Verification items for the finished model (mm, model axes). A direction names the side the tool comes from. Round coordinates to 2 decimals unless told otherwise and drop trailing zeros. Write each loop counter-clockwise with the first axis right and the second up, starting at its lowest first coordinate (ties: lowest second). Pieces come first, ordered by that corner, then holes. Notation, with made-up numbers: M 79,70.5 L 135,70.5 A20 cw 135,92.5 Z; hole C 14.25,26.25 d1. An arc over 180 degrees is marked long. One line per item, written item: value. Start each with the question number.
Item 1: Section check A-A, the plane y = -27.5. Record the cut outline in (x, z), then the cut area to 3 significant figures.
Item 2: Draft check along X on faces 4 (the face through (-1.671, -50.089, 3.473)), 5 (the face through (3.916, -98, 9)), 6 (the face through (2.498, -51, -57)), 7 (the face through (-3, -61, -50.482)). Enter one of: +X half, -X half, draft (parallel to the pull), parting line (faces both ways), or undercut.
Item 3: Section check C-C, the plane z = 12.5. Record the cut outline in (x, y).
Item 4: Gauge pin test, flat ends, axial feed: pin 1 (6 mm diameter, centred on x = 27, y = -39, fed in from +Z); pin 2 (12 mm diameter, centred on x = 29.5, y = -60, fed in from -Z); pin 3 (8 mm diameter, centred on x = -5, z = -53.5, fed in from -Y); pin 4 (1.9 mm diameter, centred on y = -98.5, z = 10, fed in from -X). Record the tip position at first contact, or that the pin passes through.
Item 5: Section check D-D, the plane x = -23.5. Record the cut outline in (y, z).
Item 6: Thickness scan on probe 1 along X at (y, z) = (-60, -20); probe 2 along X at (y, z) = (-60, -28.5); probe 3 along Z at (x, y) = (-10.5, -50). Record the ranges inside material, lowest first. Write a range as from..to.
Item 7: Section check B-B, the plane x = -2. Record the cut outline in (y, z), then the cut area to 3 significant figures.
Item 8: Tool access check on faces 1 (the face through (7, -95.25, 8)), 2 (the face through (10.266, -98, 5)), 3 (the face through (-3, -55.88, -57)). Record the directions out of +Z, -Z, +X, -X, +Y, -Y that give a thin tool (end or side, any length) a straight path to the whole face; none if there is none.
from build123d import *

# Parameters (mm, degrees)
F1_DEPTH = 101.6
F3_DEPTH = 6.35
F4_W     = 10.16
F4_H     = 10.16
F5_DEPTH = 12.7
F6_W     = 10.16
F6_H     = 10.16
F7_DEPTH = 12.7


with BuildPart() as f1:
    # F0 (on Front) → F1 (new body)
    with BuildSketch(Plane.XZ):
        Polygon((-3.390036, 1.964426), (-53.382213, -50.482459), (48.217787, -50.482459), (2.192216, 1.964426), (0, 4.939404), align=None)
    extrude(amount=F1_DEPTH)

    # F2 (on face) → F3 (join)
    with BuildSketch(Plane.XZ.offset(101.6)):
        Polygon((3.916128, 16.882844), (3.916128, 0), (10.266128, -7.235928), (10.266128, 16.882844), align=None)
    extrude(amount=-F3_DEPTH)

    # F4 (on face) → F5 (join)
    with BuildSketch(Plane(origin=(0, 0, -50.482459), x_dir=(1, 0, 0), z_dir=(0, 0, -1))):
        with Locations((-2.582213, 50.8)):
            Rectangle(F4_W, F4_H)
    extrude(amount=-F5_DEPTH)

    # F6 (on face) → F7 (join)
    with BuildSketch(Plane(origin=(0, 0, -50.482459), x_dir=(1, 0, 0), z_dir=(0, 0, -1))):
        with Locations((-2.582213, 50.8)):
            Rectangle(F6_W, F6_H)
    extrude(amount=F7_DEPTH)


solid = f1.part
Response values:
1. outline: M -53.38,-50.48 L 48.22,-50.48 L 2.19,1.96 L 0,4.94 L -3.39,1.96 Z
1. area: 2,820 mm2
2. face 4: -X half
2. face 5: undercut
2. face 6: +X half
2. face 7: draft
3. outline: M 3.92,-101.6 L 10.27,-101.6 L 10.27,-95.25 L 3.92,-95.25 Z
4. pin 1: stops at z = -22.89
4. pin 2: stops at z = -50.48
4. pin 3: stops at y = -101.6
4. pin 4: stops at x = 3.92
5. outline: M -101.6,-50.48 L 0,-50.48 L 0,-19.13 L -101.6,-19.13 Z
6. probe 1: x = -24.33..21.47
6. probe 2: x = -32.43..28.93
6. probe 3: z = -50.48..-5.49
7. outline: M -101.6,-50.48 L -55.88,-50.48 L -55.88,-63.18 L -45.72,-63.18 L -45.72,-50.48 L 0,-50.48 L 0,3.18 L -101.6,3.18 Z
7. area: 5,580 mm2
8. face 1: +Z, +X, +Y
8. face 2: +Z, +X, +Y, -Y
8. face 3: -Z, +X, -X, -Y
